```python
from build123d import *

# Parameters (mm, degrees)
BOSS_EXTRUDE1_DEPTH        = 3.175
F_1_8_0_1250_DOWEL_HOLE1_D = 3.175
SKETCH4_R                  = 4.7625
CUT_EXTRUDE1_DEPTH         = 39.125563171
M4_CLEARANCE_HOLE1_D       = 4.5


with BuildPart() as part:
    # Sketch1 → Boss-Extrude1 (new body)
    with BuildSketch(Plane(origin=(0, 0, 0), x_dir=(1, 0, 0), z_dir=(0, 1, 0))):
        with BuildLine():
            Line((4.957224307, 22.517830961), (6.192571563, 13.134436958))
            ThreePointArc((6.192571563, 13.134436958), (8.485281374, 8.485281374), (13.134436958, 6.192571563))
            Line((13.134436958, 6.192571563), (22.517830961, 4.957224307))
            ThreePointArc((22.517830961, 4.957224307), (26.8652, 0), (22.517830961, -4.957224307))
            Line((22.517830961, -4.957224307), (13.134436958, -6.192571563))
            ThreePointArc((13.134436958, -6.192571563), (10.620595205, -6.955137122), (8.485281374, -8.485281374))
            Line((8.485281374, -8.485281374), (-8.485281374, 8.485281374))
            ThreePointArc((-8.485281374, 8.485281374), (-6.955137122, 10.620595205), (-6.192571563, 13.134436958))
            Line((-6.192571563, 13.134436958), (-4.957224307, 22.517830961))
            ThreePointArc((-4.957224307, 22.517830961), (0, 26.8652), (4.957224307, 22.517830961))
        make_face()
    boss_extrude1 = extrude(amount=BOSS_EXTRUDE1_DEPTH)

    # Mirror7: Boss-Extrude1 across plane
    add(boss_extrude1.mirror(Plane(origin=(-8.485281374, 3.175, -8.485281374), x_dir=(0.7071067811865467, 0, 0.7071067811865483), z_dir=(0.7071067811865486, 0, -0.7071067811865466))))

    # 1/8 (0.1250) Dowel Hole1 (through all)
    with Locations(Plane(origin=(0, 3.175, 0), x_dir=(1, 0, 0), z_dir=(0, 1, 0))):
        with Locations((0, 21.8652), (0, -21.8652), (-21.8652, 0), (21.8652, 0)):
            Hole(F_1_8_0_1250_DOWEL_HOLE1_D / 2)

    # Sketch4 → Cut-Extrude1 (cut, through all)
    with BuildSketch(Plane(origin=(0, 3.175, 0), x_dir=(1, 0, 0), z_dir=(0, 1, 0))):
        with Locations(Location((0, 0, 0), (0, 0, 270))):
            Circle(SKETCH4_R)
    extrude(amount=-CUT_EXTRUDE1_DEPTH, mode=Mode.SUBTRACT)

    # M4 Clearance Hole1 (through all)
    with Locations(Plane(origin=(0, 3.175, 0), x_dir=(1, 0, 0), z_dir=(0, 1, 0))):
        with Locations((-11.313708499, 0), (0, 11.313708499), (11.313708499, 0), (0, -11.313708499)):
            Hole(M4_CLEARANCE_HOLE1_D / 2)


solid = part.part
```
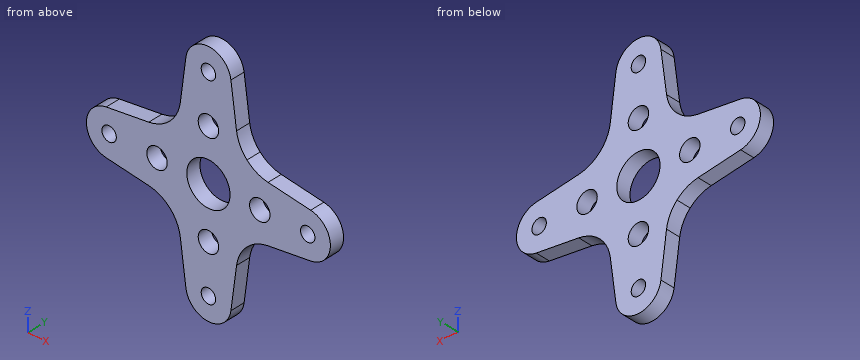
For this review, take the finished solid that the model builds, in its own axes (mm). Round coordinates to 2 decimals unless told otherwise and drop trailing zeros. Write each loop counter-clockwise with the first axis right and the second up, starting at its lowest first coordinate (ties: lowest second). Pieces come first, ordered by that corner, then holes. Notation, with made-up numbers: (-36, 30.25) - (-20, 30.25) arc R19 ccw to (-20, 35.25) - close; hole circle Ø3 at (80, 52). An arc over 180 degrees is marked (long way). Answer as CSV lines item,"result". Start each with the question number.
(1) Add section D-D, the plane y = 1.4. State how many separate pieces and enclosed holes the cut face has, plus the area to 3 significant figures.
(2) Add section B-B, the plane x = 0. State the section outline as (y, z) points (1 decimal).
(3) For pin 1 (4 mm diameter, centred on x = 21.87, z = 0, fed in from +Y) (3 decimals); pin 2 (1 mm diameter, centred on x = -11, y = 2.5, fed in from +Z), all flat-tipped, find the tip position at first contact; note any pin that passes through.
(4) Add section A-A, the plane z = 0. State the section outline as (x, y) points (1 decimal).
(5) For line 1 (Z direction, x = -12, y = 2.25); line 2 (X direction, y = 1.4, z = 11); line 3 (X direction, y = 0.3, z = -23), list the stretches that pass through material, from the lowest coordinate up.
(6) Add section C-C, the plane z = -21. State the section outline as (x, y) points (3 decimals), plus the area to 3 significant figures.
From the geometry:
1,separate pieces,"1"
1,enclosed holes,"9"
1,area,"932 mm²"
2,outline,"(0, -26.9) - (3.2, -26.9) - (3.2, -23.5) - (0, -23.5) - close; (0, -20.3) - (3.2, -20.3) - (3.2, -13.6) - (0, -13.6) - close; (0, -9.1) - (3.2, -9.1) - (3.2, -4.8) - (0, -4.8) - close; (0, 4.8) - (3.2, 4.8) - (3.2, 9.1) - (0, 9.1) - close; (0, 13.6) - (3.2, 13.6) - (3.2, 20.3) - (0, 20.3) - close; (0, 23.5) - (3.2, 23.5) - (3.2, 26.9) - (0, 26.9) - close"
3,pin 1,"stops at y = 3.175"
3,pin 2,"stops at z = 7.02"
4,outline,"(-26.9, 0) - (-23.5, 0) - (-23.5, 3.2) - (-26.9, 3.2) - close; (-20.3, 0) - (-13.6, 0) - (-13.6, 3.2) - (-20.3, 3.2) - close; (-9.1, 0) - (-4.8, 0) - (-4.8, 3.2) - (-9.1, 3.2) - close; (4.8, 0) - (9.1, 0) - (9.1, 3.2) - (4.8, 3.2) - close; (13.6, 0) - (20.3, 0) - (20.3, 3.2) - (13.6, 3.2) - close; (23.5, 0) - (26.9, 0) - (26.9, 3.2) - (23.5, 3.2) - close"
5,line 1,"z = -6.43 to -2.14, 2.14 to 6.43"
5,line 2,"x = -6.78 to -2.23, 2.23 to 6.78"
5,line 3,"x = -4.87 to -1.11, 1.11 to 4.87"
6,outline,"(-5.157, 0) - (-1.331, 0) - (-1.331, 3.175) - (-5.157, 3.175) - close; (1.331, 0) - (5.157, 0) - (5.157, 3.175) - (1.331, 3.175) - close"
6,area,"24.3 mm²"
